Geometry check sheet. Reference: the model listing, model coordinates, mm. A direction names the side the tool comes from. Coordinates: 2 decimals unless noted, no trailing zeros. Write each loop counter-clockwise with the first axis right and the second up, starting at its lowest first coordinate (ties: lowest second). Pieces come first, ordered by that corner, then holes. Notation, with made-up numbers: (87, 24.5) -> (135, 24.5) arc R28 cw to (135, 42.5) -> close; hole circle Ø8 at (-14.75, -15.5). An arc over 180 degrees is marked (long way). One line per question, with ' | ' between items.
```python
from build123d import *

# Parameters (mm, degrees)
PAD_DEPTH       = 6
SKETCH001_R     = 4
POCKET_DEPTH    = 6.001
SKETCH002_W     = 27
SKETCH002_H     = 8
PAD001_DEPTH    = 2.3
SKETCH003_R     = 2.6
POCKET001_DEPTH = 2.301


with BuildPart() as part:
    # Sketch → Pad (new body)
    with BuildSketch(Plane.XY):
        with BuildLine():
            Line((-12.5, 6.5), (12.5, 6.5))
            ThreePointArc((13.5, 5.5), (13.207107, 6.207107), (12.5, 6.5))
            Line((13.5, 5.5), (13.5, -5.5))
            ThreePointArc((12.5, -6.5), (13.207107, -6.207107), (13.5, -5.5))
            Line((12.5, -6.5), (-12.5, -6.5))
            ThreePointArc((-13.5, -5.5), (-13.207107, -6.207107), (-12.5, -6.5))
            Line((-13.5, -5.5), (-13.5, 5.5))
            ThreePointArc((-12.5, 6.5), (-13.207107, 6.207107), (-13.5, 5.5))
        make_face()
    extrude(amount=PAD_DEPTH)

    # Sketch001 (on Face10 of Pad) → Pocket (cut, through all)
    with BuildSketch(Plane.XY.offset(6)):
        with Locations((-5.1, 0)):
            Circle(SKETCH001_R)
        with Locations((5.1, 0)):
            Circle(SKETCH001_R)
    extrude(amount=-POCKET_DEPTH, mode=Mode.SUBTRACT)

    # Sketch002 (on Face5 of Pocket) → Pad001 (join)
    with BuildSketch(Plane.XY.offset(6)):
        Rectangle(SKETCH002_W, SKETCH002_H)
    extrude(amount=PAD001_DEPTH)

    # Sketch003 (on Face18 of Pad001) → Pocket001 (cut, through all)
    with BuildSketch(Plane(origin=(0, 0, 6), x_dir=(1, 0, 0), z_dir=(0, 0, -1))):
        with Locations((-5.1, 0)):
            Circle(SKETCH003_R)
        with Locations((5.1, 0)):
            Circle(SKETCH003_R)
    extrude(amount=-POCKET001_DEPTH, mode=Mode.SUBTRACT)


solid = part.part
```
(1) Tool access check on faces 1 (the face through (-13.199, 6.215, 2.958)), 2 (the face through (-2, 0, 6)), 3 (the face through (0, -4, 7)), 4 (the face through (0, 5, 6)), 5 (the face through (0, 0, 0)). Record the directions out of +Z, -Z, +X, -X, +Y, -Y that give a thin tool (end or side, any length) a straight path to the whole face; none if there is none.
Answers below:
face 1: +Z, -Z, -X, +Y | face 2: -Z | face 3: +Z, +X, -X, -Y | face 4: +Z, +X, -X, +Y | face 5: -Z, +X, -X, +Y, -Y
(2) Cross-section at A-A (z = 7). Record the cut outline in (x, y).
Answers below:
outline: (-13.5, -4) -> (13.5, -4) -> (13.5, 4) -> (-13.5, 4) -> close; hole circle Ø5.2 at (-5.1, 0); hole circle Ø5.2 at (5.1, 0)
(3) Cross-section at D-D (z = 4.25). Record the cut outline in (x, y), plus the area to 3 significant figures.
Answers below:
outline: (-13.5, -5.5) arc R1 ccw to (-12.5, -6.5) -> (12.5, -6.5) arc R1 ccw to (13.5, -5.5) -> (13.5, 5.5) arc R1 ccw to (12.5, 6.5) -> (-12.5, 6.5) arc R1 ccw to (-13.5, 5.5) -> close; hole circle Ø8 at (-5.1, 0); hole circle Ø8 at (5.1, 0) | area: 250 mm²
(4) Material ranges on line 1 (X direction, y = 0, z = 6.65); line 2 (X direction, y = 0, z = 2.85); line 3 (Y direction, x = -5.1, z = 7.75), recorded low to high.
Answers below:
line 1: x = -13.5 to -7.7, -2.5 to 2.5, 7.7 to 13.5 | line 2: x = -13.5 to -9.1, -1.1 to 1.1, 9.1 to 13.5 | line 3: y = -4 to -2.6, 2.6 to 4
(5) Depth check by flat-ended pin: P1, Ø3, axis at x = -5.1, y = 0, coming from the -Z side; P2, Ø6.5, axis at x = 5.5, y = 0.5, coming from the -Z side; P3, Ø2.5, axis at x = -3, z = 7.5, coming from the +Y side; P4, Ø2, axis at x = -4.5, y = 6, coming from the +Z side. Enter the tip coordinate at first touch or a pass-through.
Answers below:
P1: passes through | P2: stops at z = 6 | P3: stops at y = 4 | P4: stops at z = 6
(6) Cross-section at C-C (x = -10.5). Record the cut outline in (y, z), plus the area to 3 significant figures.
Answers below:
outline: (-6.5, 0) -> (6.5, 0) -> (6.5, 6) -> (4, 6) -> (4, 8.3) -> (-4, 8.3) -> (-4, 6) -> (-6.5, 6) -> close | area: 96.4 mm²
(7) Draft check along Y on faces 6 (the face through (13.199, -6.215, 2.958)), 7 (the face through (7.58, -0.78, 7.13)), 8 (the face through (0, -5, 6)), 9 (the face through (-2.62, -0.78, 7.13)). Enter one of: pulls with the +Y half, pulls with the -Y half, needs draft (parallel to the pull), parting line crosses it, or undercut.
Answers below:
face 6: pulls with the -Y half | face 7: undercut | face 8: needs draft | face 9: undercut
(8) Cross-section at B-B (y = 0). Record the cut outline in (x, z), plus the area to 3 significant figures.
Answers below:
outline: (-13.5, 0) -> (-9.1, 0) -> (-9.1, 6) -> (-7.7, 6) -> (-7.7, 8.3) -> (-13.5, 8.3) -> close; (-2.5, 6) -> (-1.1, 6) -> (-1.1, 0) -> (1.1, 0) -> (1.1, 6) -> (2.5, 6) -> (2.5, 8.3) -> (-2.5, 8.3) -> close; (7.7, 6) -> (9.1, 6) -> (9.1, 0) -> (13.5, 0) -> (13.5, 8.3) -> (7.7, 8.3) -> close | area: 104 mm²
